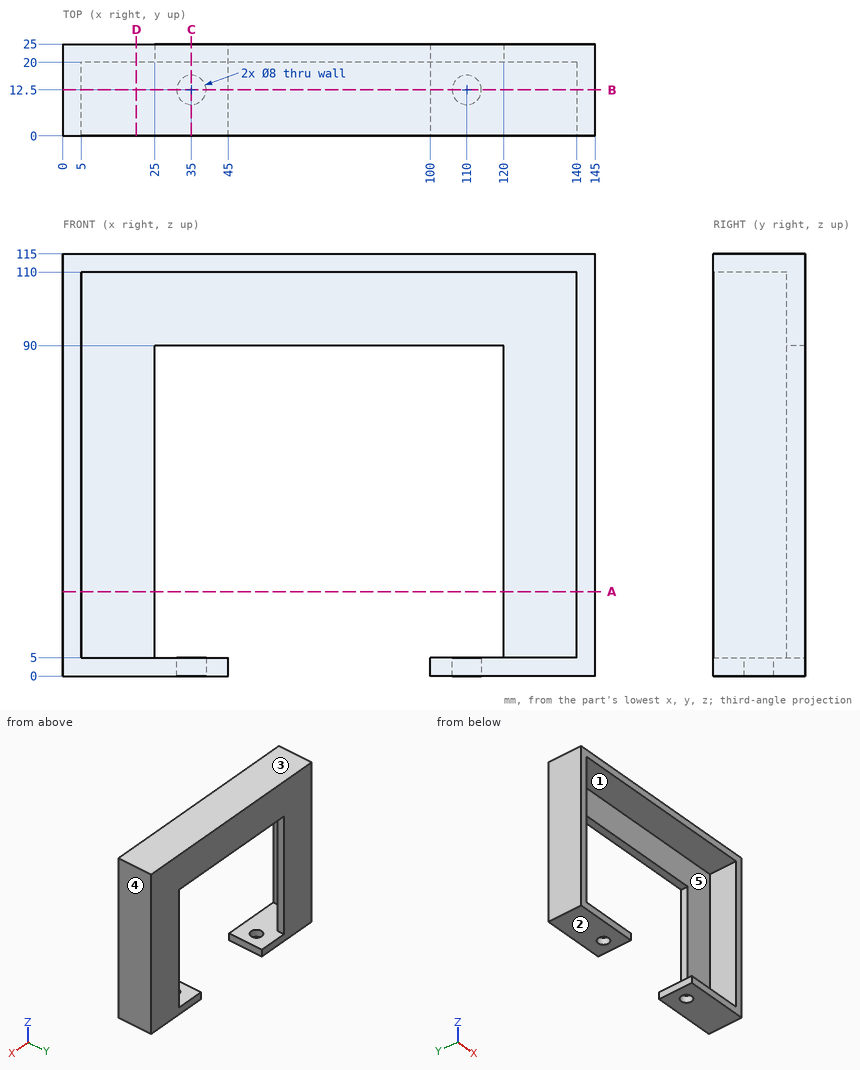
Print and shaded views of the part. All mm, measured from the part's lowest x, y and z. A direction names the side the tool comes from. Round coordinates to 2 decimals unless told otherwise and drop trailing zeros. Loops run counter-clockwise (first coordinate to the right, second up) from the corner with the lowest first, then second, coordinate; pieces in that order, holes last. Notation, with made-up numbers: M 39.5,11.5 L 94.5,11.5 A19 ccw 94.5,45.5 Z; hole C 31.5,59.5 d3. An arc over 180 degrees is marked long. One line per question, with ' | ' between items.
1) Band-saw the part on B-B (y = 12.5). Give the cut face in (x, z).
Solved:
outline: M 0,0 L 31,0 L 31,5 L 5,5 L 5,110 L 140,110 L 140,5 L 114,5 L 114,0 L 145,0 L 145,115 L 0,115 Z; M 39,0 L 45,0 L 45,5 L 39,5 Z; M 100,0 L 106,0 L 106,5 L 100,5 Z
2) Band-saw the part on A-A (z = 23). Give the cut face in (x, y), then the cut area to 3 significant figures.
Solved:
outline: M 0,0 L 5,0 L 5,20 L 25,20 L 25,25 L 0,25 Z; M 120,20 L 140,20 L 140,0 L 145,0 L 145,25 L 120,25 Z | area: 450 mm²
3) Mould opens along X. For the marked faces 3, 4 and 5 say: +X half, -X half, draft (parallel to the pull), parting line (faces both ways), or undercut.
Solved:
face 3: draft | face 4: +X half | face 5: undercut
4) Band-saw the part on D-D (x = 20). Give the cut face in (y, z), then the cut area to 3 significant figures.
Solved:
outline: M 0,0 L 25,0 L 25,115 L 0,115 L 0,110 L 20,110 L 20,5 L 0,5 Z | area: 775 mm²
5) 3-axis set-ups, long thin cutter, end or side, ignore diameter. For the marked faces 1 and 2: which of +Z, -Z, +X, -X, +Y, -Y reach the whole face in a straight line?
Solved:
face 1: -Y | face 2: -Z, +X, -X, +Y, -Y
6) Flat gauge pins, fed straight in: pin 1 (6.5 mm diameter, centred on x = 35, y = 12.5, fed in from -Z); pin 2 (10 mm diameter, centred on x = 78, y = 21, fed in from -Z). Where does each tip first touch, or does it go through?
Solved:
pin 1: stops at z = 110 | pin 2: stops at z = 90
7) Drill centre lines: line 1 along Z through (x, y) = (119, 4); line 2 along Y through (x, z) = (35, 1.25); line 3 along X through (y, z) = (16.75, 78). Where is each one in solid material? Low to high.
Solved:
line 1: z = 0 to 5, 110 to 115 | line 2: y = 0 to 8.5, 16.5 to 25 | line 3: x = 0 to 5, 140 to 145
8) Band-saw the part on C-C (x = 35). Give the cut face in (y, z), then the cut area to 3 significant figures.
Solved:
outline: M 0,0 L 8.5,0 L 8.5,5 L 0,5 Z; M 0,110 L 20,110 L 20,90 L 25,90 L 25,115 L 0,115 Z; M 16.5,0 L 25,0 L 25,5 L 16.5,5 Z | area: 310 mm²
